```python
from build123d import *

# Parameters (mm, degrees)
SKETCH2_R               = 2.5
CUT_EXTRUDE1_DEPTH      = 6
CUT_EXTRUDE1_DEPTH_BACK = 6
SKETCH4_W               = 12
SKETCH4_H               = 18
CUT_EXTRUDE2_DEPTH      = 1.830127
SKETCH3_R               = 3
SKETCH3_R_2             = 2.5
EXTRUDE_THIN1_DEPTH     = 3.75


with BuildPart() as part:
    # Sketch1 → Revolve1 (revolve)
    with BuildSketch(Plane.XY):
        with BuildLine():
            Line((0, 0), (0, -7))
            Line((0, -7), (1.75, -7))
            Line((1.75, -7), (1.75, -17))
            Line((1.75, -17), (3.5, -17))
            Line((3.5, -17), (3.5, -3.570714214))
            ThreePointArc((3.5, -3.570714214), (4.628907596, 1.890294809), (0, 5))
            Line((0, 5), (0, 0))
        make_face()
    revolve(axis=Axis((0, 0, 0), (0, 1, 0)))

    # Sketch2 → Cut-Extrude1 (cut, two sides)
    with BuildSketch(Plane.XY) as cut_extrude1_sk:
        Circle(SKETCH2_R)
    extrude(amount=CUT_EXTRUDE1_DEPTH, mode=Mode.SUBTRACT)
    extrude(cut_extrude1_sk.sketch, amount=-CUT_EXTRUDE1_DEPTH_BACK, mode=Mode.SUBTRACT)

    # Sketch4 → Cut-Extrude2 (cut)
    with BuildSketch(Plane.XY.offset(2.5)):
        Rectangle(SKETCH4_W, SKETCH4_H)
    cut_extrude2 = extrude(amount=CUT_EXTRUDE2_DEPTH, mode=Mode.SUBTRACT)

    # Mirror1: Cut-Extrude2 across plane
    add(cut_extrude2.mirror(Plane.XY), mode=Mode.SUBTRACT)

    # Sketch3 → Extrude-Thin1 (add, symmetric)
    with BuildSketch(Plane.XY):
        Circle(SKETCH3_R)
        Circle(SKETCH3_R_2, mode=Mode.SUBTRACT)
    extrude(amount=EXTRUDE_THIN1_DEPTH, both=True)

    # Mirror2: part across plane


with BuildPart() as part_1:
    add(part.part)
    add(part.part.mirror(Plane(origin=(1.75, -17, 0), x_dir=(0, 0, 1), z_dir=(0, -1, 0))))


solid = part_1.part
```
Verification items for the finished model (mm, model axes). A direction names the side the tool comes from. Round coordinates to 2 decimals unless told otherwise and drop trailing zeros. Loops run counter-clockwise (first coordinate to the right, second up) from the corner with the lowest first, then second, coordinate; pieces in that order, holes last. Notation, with made-up numbers: (-7.5, -13.75) -> (45.5, -13.75) arc R25 cw to (45.5, 16.25) -> close; hole circle Ø10 at (10.5, -13.5). An arc over 180 degrees is marked (long way). Answer as a JSON object with one key per item and string values.
Q1. Go/stop test with flat-tipped pins: P1, Ø3, axis at x = -1.5, z = 2, coming from the +Y side; P2, Ø3, axis at x = 1, z = -2.5, coming from the -Y side; P3, Ø0.5, axis at x = 0.5, z = -3, coming from the +Y side; P4, Ø4, axis at x = -0.5, z = -0.5, coming from the -Y side. Record where each tip stops, or that it passes through.
Data:
{"P1": "stops at y = 4.9", "P2": "stops at y = -38.86", "P3": "stops at y = 2.99", "P4": "stops at y = -39"}
Q2. Section check B-B (z = 0). Record the boundary of the cut face in (x, y), then the cut area to 3 significant figures.
Data:
{"outline": "(-3.5, -30.43) arc R5 ccw (long way) to (3.5, -30.43) -> (3.5, -3.57) arc R5 ccw (long way) to (-3.5, -3.57) -> close; hole circle Ø5 at (0, -34); hole circle Ø5 at (0, 0); hole (-1.75, -27) -> (1.75, -27) -> (1.75, -7) -> (-1.75, -7) -> close", "area": "222 mm2"}
Q3. Access from +Z, -Z, +X, -X, +Y, -Y to the whole of each face (thin tool, end or side, straight path). Record for faces 4 (the flat face through (0, -25, -3)), 5 (the flat face through (0, -25, 3)), 6 (the cylindrical face through (-3.497, -17.188, -0.154)), 7 (the cylindrical face through (-3, 0, -3)).
Data:
{"face 4": "-Z, +X, -X", "face 5": "+Z, +X, -X", "face 6": "none", "face 7": "-Z"}
Q4. Scan lines: line 1 (X direction, y = -9, z = 0); line 2 (Y direction, x = 1, z = 0.25); line 3 (Y direction, x = 0, z = -0.5). Record each from-to range of solid material in increasing order. Write a range as from..to.
Data:
{"line 1": "x = -3.5..-1.75, 1.75..3.5", "line 2": "y = -38.89..-36.29, -31.71..-27, -7..-2.29, 2.29..4.89", "line 3": "y = -38.97..-36.5, -31.5..-27, -7..-2.5, 2.5..4.97"}
Q5. Section check D-D (y = -18). Record the boundary of the cut face in (x, z), then the cut area to 3 significant figures.
Data:
{"outline": "circle Ø7 at (0, 0); hole circle Ø3.5 at (0, 0)", "area": "28.9 mm2"}
Q6. Section check C-C (x = 0). State how many separate pieces and enclosed holes the cut face has, then the cut area to 3 significant figures.
Data:
{"separate pieces": "3", "enclosed holes": "1", "area": "135 mm2"}
Q7. Section check A-A (y = -34). Record the boundary of the cut face in (x, z), then the cut area to 3 significant figures.
Data:
{"outline": "(-4.33, -2.5) -> (-3, -2.5) -> (-3, -3.75) -> (-2.5, -3.75) -> (-2.5, 3.75) -> (-3, 3.75) -> (-3, 2.5) -> (-4.33, 2.5) arc R5 ccw to start; (2.5, -3.75) -> (3, -3.75) -> (3, -2.5) -> (4.33, -2.5) arc R5 ccw to (4.33, 2.5) -> (3, 2.5) -> (3, 3.75) -> (2.5, 3.75) -> close", "area": "25.3 mm2"}
Q8. Draft check along Y on faces 1 (the flat face through (0, -30, 2.5)), 2 (the flat face through (-2, 2, -3.75)), 3 (the cylindrical face through (-0.54, -2.44, -0.05)). Enter one of: pulls with the +Y half, pulls with the -Y half, needs draft (parallel to the pull), parting line crosses it, or undercut.
Data:
{"face 1": "undercut", "face 2": "needs draft", "face 3": "undercut"}
